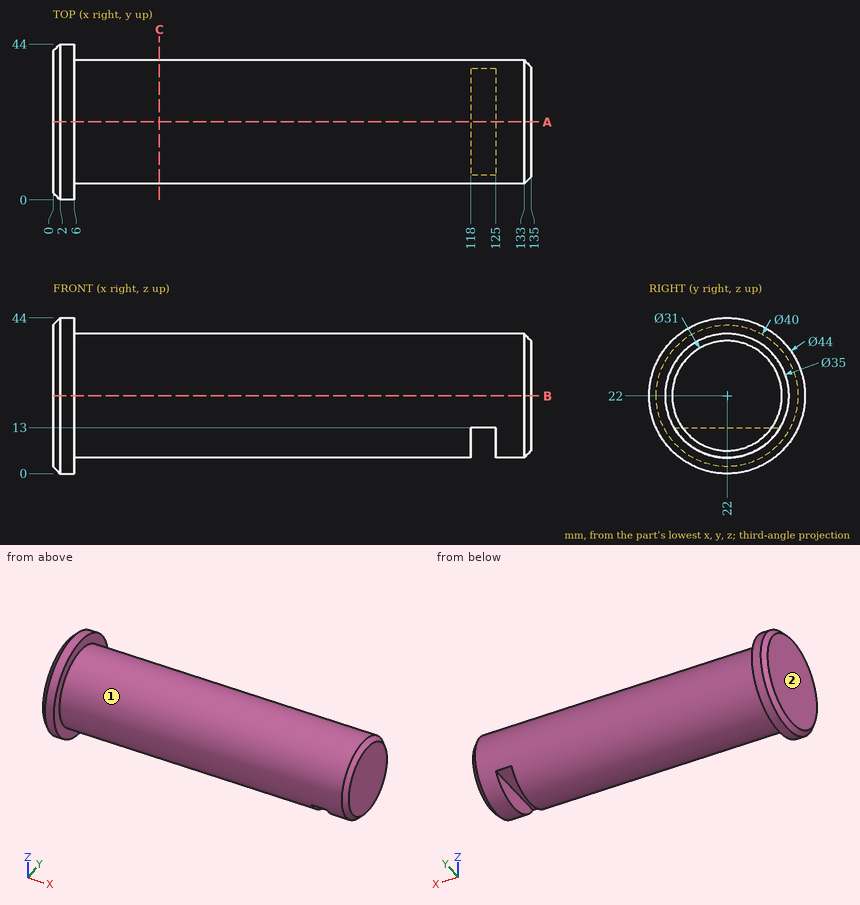
Verification items for this drawing (mm, ordinates from the low corner). A direction names the side the tool comes from. Give positions to 0.01 mm unless a question says otherwise; leave off trailing zeros. Order: outer loops, then holes, each group sorted by start corner. A loop starts at its lowest first (then second) coordinate and runs counter-clockwise, first axis right, second up.
1) Cross-section at C-C (x = 30). Record the boundary of the cut face in (y, z).
Results are:
outline: circle Ø35 at (22, 22)
2) Gauge pin test, flat ends, axial feed: pin 1 (1 mm diameter, centred on x = 85, z = 31, fed in from -Y); pin 2 (6 mm diameter, centred on x = 114.5, z = 11, fed in from -Y); pin 3 (10 mm diameter, centred on x = 37, y = 24, fed in from -Z). Record the tip position at first contact, or that the pin passes through.
Results are:
pin 1: stops at y = 6.7
pin 2: stops at y = 6.44
pin 3: stops at z = 4.5
3) Material ranges on probe 1 along X at (y, z) = (33, 12.5); probe 2 along X at (y, z) = (35, 12); probe 3 along Z at (x, y) = (75.5, 31), recorded low to high.
Results are:
probe 1: x = 0 to 118, 125 to 135
probe 2: x = 0 to 118, 125 to 134.1
probe 3: z = 6.99 to 37.01
4) Tool access check on the marked faces 1 and 2. Record the directions out of +Z, -Z, +X, -X, +Y, -Y that give a thin tool (end or side, any length) a straight path to the whole face; none if there is none.
Results are:
face 1: +X
face 2: +Z, -Z, -X, +Y, -Y
5) Cross-section at B-B (z = 22). Record the boundary of the cut face in (x, y), then the cut area to 3 significant figures.
Results are:
outline: (0, 2) - (2, 0) - (6, 0) - (6, 4.5) - (133, 4.5) - (135, 6.5) - (135, 37.5) - (133, 39.5) - (6, 39.5) - (6, 44) - (2, 44) - (0, 42) - close
area: 4,770 mm2
6) Cross-section at A-A (y = 22). Record the boundary of the cut face in (x, z).
Results are:
outline: (0, 2) - (2, 0) - (6, 0) - (6, 4.5) - (118, 4.5) - (118, 13) - (125, 13) - (125, 4.5) - (133, 4.5) - (135, 6.5) - (135, 37.5) - (133, 39.5) - (6, 39.5) - (6, 44) - (2, 44) - (0, 42) - close
